Autodesk Inventor part; units mm, degrees
ref_plane "Work Plane1" through (1.525, 0, 0) normal (0, 0, 1) x (1, 0, 0)
ref_plane "YZ Plane" through (0, 0, 0) normal (1, 0, 0) x (0, 1, 0)
ref_plane "XZ Plane" through (0, 0, 0) normal (0, 1, 0) x (-1, 0, 0)
sketch "Skizze1" plane through (0, 0, 0) normal (0, 0, 1) x (1, 0, 0)
  line L0 (0, 6) -> (55, 6)
  line L1 (55, 6) -> (55, 0)
  line L2 (55, 0) -> (0, 0)
  line L3 (-11, 0) -> (66, 0)
  line L4 (0, -1.2) -> (0, 7.2)
  line L5 (0, 6) -> (0, 0)
  dimension "d2" = 12
  dimension "d59" = 55
revolve "Körper" add sketch "Skizze1" angle 360 about axis through (55, 0, 0) along (-1, 0, 0)
sketch "Skizze2" plane through (0, 0, 0) normal (-1, 0, 0) x (0, 0, 1)
  line L0 (0, 9.815) -> (8.5, 4.9075)
  line L1 (8.5, 4.9075) -> (8.5, -4.9075)
  line L2 (8.5, -4.9075) -> (0, -9.815)
  line L3 (0, -9.815) -> (-8.5, -4.9075)
  line L4 (-8.5, -4.9075) -> (-8.5, 4.9075)
  line L5 (-8.5, 4.9075) -> (0, 9.815)
  line L6 (-11.9, 0) -> (11.9, 0)
  line L7 (0, 13.7409) -> (0, -13.7409)
  point P0 (0, 0)
  point P1 (0, 0)
  dimension "d11" = 17
extrude "Kopf" add sketch "Skizze2" along normal blind 7.5
sketch "Skizze4" plane through (0, 0, 0) normal (0, 0, 1) x (1, 0, 0)
  line L0 (-6.5185, 10.2) -> (-7.5, 8.5)
  line L1 (-1.1, 0) -> (-0.234, 0)
  line L2 (-8.9532, 0) -> (1.2192, 0)
  line L3 (-7.5, 10.2) -> (-6.5185, 10.2)
  line L4 (-7.5, 8.5) -> (-7.5, 10.2)
  line L5 (0, 12.24) -> (0, -2.04)
  dimension "d65" = 17
  dimension "d67" = 30
  dimension "d68" = 20.4
  dimension "d69" = 7.5
revolve "Fase1" cut sketch "Skizze4" angle 360 about axis through (-1.1, 0, 0) along (1, 0, 0)
thread "Gewinde"
chamfer "Fase2" distance 1.0735 distance2 1.0736 1 edges at (55, -6, 0) measured on face at (55, 1.497, -1.3262)
fillet "Fillet2" radius 0.1 1 edges at (0, -6, 0)
ref_plane "Work Plane1" through (1.525, 0, 0) normal (0, 0, 1) x (1, 0, 0)
equation "\"d2\" = GD"
equation "\"d59\" = NLG"
equation "\"d11\" = SW"
equation "\"d3\" = KOH"
equation "\"d71\" = RR"
equation "\"d15\" = GEL"
equation "\"d6\" = -0.5 * SPD + 0.5 * GD"
equation "\"d65\" = SW"
equation "\"d67\" = ANG1"
equation "\"d68\" = 1.2 * SW"
equation "\"d69\" = KOH"
equation "\"NLG\" = 55"
equation "\"GD\" = NND"
equation "\"BDM\" = NND"
equation "\"KOH\" = 7.5"
equation "\"GEL\" = 30"
equation "\"SW\" = 17"
equation "\"SW0\" = SW"
equation "\"SPD\" = NND - 1.2269 * PTC"
equation "\"SD2\" = NND"
equation "\"SD\" = 0"
equation "\"ANG1\" = 30deg"
equation "\"GAL\" = 0.61345 * PTC"
equation "\"GUL\" = 0.61345 * PTC"
equation "\"RR\" = 0.1"
equation "\"RR1\" = 0.1"
equation "\"GD1\" = THREADDIA - 1.2269 * PTC"
equation "\"THREADDIA\" = 12"
equation "\"TOA\" = 30deg"
equation "\"PTC\" = 1.75"
equation "\"NND\" = 12"
equation "\"E0\" = 1.155 * SW"
properties part number "ISO 4016 - M12 x 55" material "Steel, Mild"
Build history of the part. All positions in model axes, mm. A direction names the side the tool comes from. Round coordinates to 2 decimals unless told otherwise and drop trailing zeros. Loops run counter-clockwise (first coordinate to the right, second up) from the corner with the lowest first, then second, coordinate; pieces in that order, holes last.
Item 1: Pin check, flat tips, straight feed: P1, Ø4, axis at x = 45.5, y = -3, coming from the -Z side; P2, Ø3, axis at x = 44, y = -4, coming from the +Z side; P3, Ø1.5, axis at x = 21, y = 0.5, coming from the -Z side. Stop position of each tip, or through.
Item 2: Drill centre lines: line 1 along X through (y, z) = (-6.5, -3.75); line 2 along Y through (x, z) = (4.5, 0.25). Where is each one in solid material? Low to high.
Item 3: Which spindle directions (+Z, -Z, +X, -X, +Y, -Y) get a long thin tool onto all of the face, cutting with end or side? Do faces 1 (the face through (-7.5, 0, 0)), 2 (the face through (0, -2, -6)). Say none if no direction does.
Item 4: Saw through at A-A (x = 8.5). List the corners of the cut face in (y, z).
Worked answers:
1. P1: stops at z = -5.92
1. P2: stops at z = 5.45
1. P3: stops at z = -6
2. line 1: x = -7.5 to 0
2. line 2: y = -5.99 to 5.99
3. face 1: +Z, -Z, -X, +Y, -Y
3. face 2: +X
4. outline: circle Ø12 at (0, 0)
